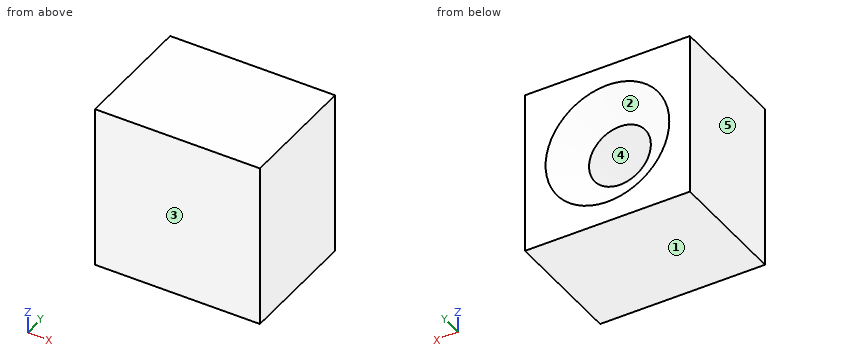
```python
from build123d import *

# Parameters (mm, degrees)
SKETCH1_W           = 80
SKETCH1_H           = 80
BOSS_EXTRUDE1_DEPTH = 60


with BuildPart() as part:
    # Sketch1 → Boss-Extrude1 (new body)
    with BuildSketch(Plane(origin=(0, 0, 0), x_dir=(1, 0, 0), z_dir=(0, 1, 0))):
        Rectangle(SKETCH1_W, SKETCH1_H)
    extrude(amount=BOSS_EXTRUDE1_DEPTH)

    # Sketch2 → Cut-Revolve1 (revolve, cut)
    with BuildSketch(Plane.XY):
        Polygon((0, 60), (-30, 60), (-15, 50), (-15, 10), (0, 10), align=None)
    revolve(axis=Axis((0, 10, 0), (0, 1, 0)), mode=Mode.SUBTRACT)


solid = part.part
```
Check sheet for the modelled part. Datum: model origin and axes. Units: mm. Face numbers are marked on the shaded views. A direction names the side the tool comes from. Round coordinates to 2 decimals unless told otherwise and drop trailing zeros. Write each loop counter-clockwise with the first axis right and the second up, starting at its lowest first coordinate (ties: lowest second). Pieces come first, ordered by that corner, then holes. Notation, with made-up numbers: M 84,-34.5 L 139,-34.5 A16 ccw 139,-7.5 Z; hole C 53.25,-18.75 d9. An arc over 180 degrees is marked long. Write item = value, one per line. Start each with the question number.
1. Release check for a two-part mould opening along Z. For the marked faces 1, 2 and 3 record: pulls with the +Z half, pulls with the -Z half, needs draft (parallel to the pull), parting line crosses it, or undercut.
2. Scan lines: line 1 (Z direction, x = 0, y = 41); line 2 (X direction, y = 30, z = -13); line 3 (X direction, y = 57, z = -15). Record each from-to range of solid material in increasing order. Write a range as [from, to].
3. Section check B-B, the plane x = 0. Record the cut outline in (y, z).
4. Section check A-A, the plane y = 33. Record the cut outline in (x, z), then the cut area to 3 significant figures.
5. Gauge pin test, flat ends, axial feed: pin 1 (2 mm diameter, centred on x = 12.5, z = 2, fed in from +Y); pin 2 (5 mm diameter, centred on x = 25, z = 8, fed in from -Y); pin 3 (1 mm diameter, centred on x = 6, z = 16.5, fed in from +Y); pin 4 (5 mm diameter, centred on x = 19, z = 19, fed in from +Y). Record the tip position at first contact, or that the pin passes through.
6. Section check C-C, the plane z = 0. Record the cut outline in (x, y), then the cut area to 3 significant figures.
7. Tool access check on the marked faces 4 and 5. Record the directions out of +Z, -Z, +X, -X, +Y, -Y that give a thin tool (end or side, any length) a straight path to the whole face; none if there is none.
Results found:
q1.face_1 = pulls with the -Z half
q1.face_2 = undercut
q1.face_3 = needs draft
q2.line_1 = [-40, -15], [15, 40]
q2.line_2 = [-40, -7.48], [7.48, 40]
q2.line_3 = [-40, -20.62], [20.62, 40]
q3.outline = M 0,-40 L 60,-40 L 60,-30 L 50,-15 L 10,-15 L 10,15 L 50,15 L 60,30 L 60,40 L 0,40 Z
q4.outline = M -40,-40 L 40,-40 L 40,40 L -40,40 Z; hole C 0,0 d30
q4.area = 5,690 mm^2
q5.pin_1 = 10
q5.pin_2 = 0
q5.pin_3 = 52.04
q5.pin_4 = 59.58
q6.outline = M -40,0 L 40,0 L 40,60 L 30,60 L 15,50 L 15,10 L -15,10 L -15,50 L -30,60 L -40,60 Z
q6.area = 3,150 mm^2
q7.face_4 = +Y
q7.face_5 = +Z, -Z, -X, +Y, -Y
